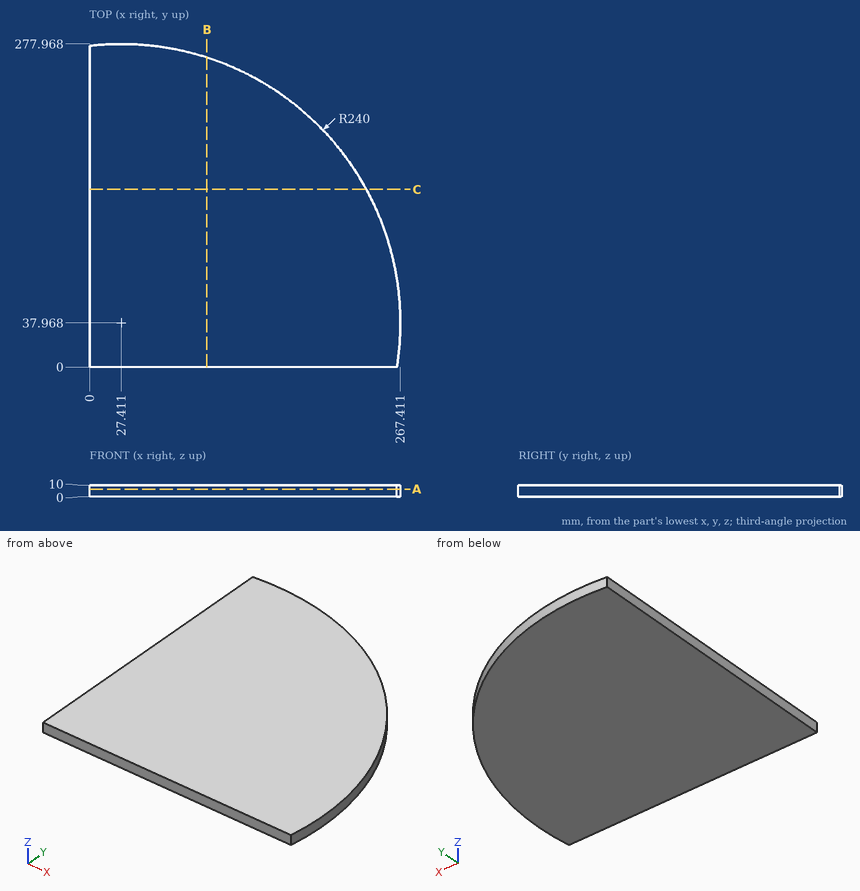
Geometry: see drawing. Coordinates: mm, zero at the bounding-box minimum. Give positions to 0.01 mm unless a question says otherwise; leave off trailing zeros. Loops run counter-clockwise (first coordinate to the right, second up) from the corner with the lowest first, then second, coordinate; pieces in that order, holes last. Notation, with made-up numbers: (84, 42) - (117, 42) arc R9 ccw to (117, 47) - close; hole circle Ø7 at (-37, -22). An arc over 180 degrees is marked (long way). Use CSV: the item, a comma, the result in double quotes. Start each with the question number.
Item 1: Section A-A on z = 6.5. Return loops of the section in (x, y), then the cut area to 3 significant figures.
Item 2: Section C-C on y = 153. Return loops of the section in (x, z).
Item 3: Line query: line 1 (Y direction, x = 237, z = 8); line 2 (X direction, y = 46.5, z = 5.5); line 3 (Y direction, x = 89.5, z = 6.25). Output: solid intervals per line, ascending.
Item 4: Section B-B on x = 101. Return loops of the section in (y, z).
Ans:
1,outline,"(0, 0) - (264.39, 0) arc R240 ccw to (0, 276.4) - close"
1,area,"61,900 mm2"
2,outline,"(0, 0) - (238.05, 0) - (238.05, 10) - (0, 10) - close"
3,line 1,"y = 0 to 154.9"
3,line 2,"x = 0 to 267.26"
3,line 3,"y = 0 to 269.8"
4,outline,"(0, 0) - (266.41, 0) - (266.41, 10) - (0, 10) - close"
